from build123d import *

# Parameters (mm, degrees)
SKETCH1_R               = 15
SKETCH1_R_2             = 10
BOSS_EXTRUDE1_DEPTH     = 125
SKETCH2_R               = 15
BOSS_EXTRUDE2_DEPTH     = 40
SKETCH11_W              = 5
SKETCH11_H              = 20
BOSS_EXTRUDE6_DEPTH     = 100
FILLET1_R               = 10
SKETCH12_W              = 28.03455484
SKETCH12_H              = 2
BOSS_EXTRUDE7_DEPTH     = 30
CUT_EXTRUDE1_DEPTH      = 23
CUT_EXTRUDE1_DEPTH_BACK = 5
SKETCH16_R              = 6.25
CUT_EXTRUDE2_DEPTH      = 7


with BuildPart() as part:
    # Sketch1 → Boss-Extrude1 (new body)
    with BuildSketch(Plane.XY):
        Circle(SKETCH1_R)
        Circle(SKETCH1_R_2, mode=Mode.SUBTRACT)
    extrude(amount=BOSS_EXTRUDE1_DEPTH)

    # Sketch2 → Boss-Extrude2 (add)
    with BuildSketch(Plane(origin=(0, 0, 0), x_dir=(1, 0, 0), z_dir=(0, 1, 0))):
        with Locations((0, -62.5)):
            Circle(SKETCH2_R)
    extrude(amount=BOSS_EXTRUDE2_DEPTH)

    # Sketch11 → Boss-Extrude6 (add)
    with BuildSketch(Plane(origin=(0, 0, 0), x_dir=(0, 0, -1), z_dir=(1, 0, 0))):
        with Locations((-62.5, 0)):
            Rectangle(SKETCH11_W, SKETCH11_H)
    extrude(amount=-BOSS_EXTRUDE6_DEPTH)

    # Fillet1
    fillet1_edges = [part.edges().sort_by_distance(p)[0] for p in [
        (-100, -10, 62.5),
        (-100, 10, 62.5),
    ]]
    fillet(fillet1_edges, radius=FILLET1_R - 0.0001)  # a hair under: the kernel refuses the full size

    # Sketch12 → Boss-Extrude7 (add)
    with BuildSketch(Plane(origin=(0, 0, 60), x_dir=(-1, 0, 0), z_dir=(0, 0, -1))):
        with Locations((28.01727742, 0)):
            Rectangle(SKETCH12_W, SKETCH12_H)
    extrude(amount=BOSS_EXTRUDE7_DEPTH)

    # Sketch13 → Cut-Extrude1 (cut, two sides: drawn at the far end of the back side and taken through both)
    with BuildSketch(Plane(origin=(0, 0, 0), x_dir=(1, 0, 0), z_dir=(0, 1, 0)).offset(-CUT_EXTRUDE1_DEPTH_BACK)):
        Polygon((-14.966629547, -30), (-42.03455484, -60), (-42.03455484, -30), align=None)
    extrude(amount=CUT_EXTRUDE1_DEPTH + CUT_EXTRUDE1_DEPTH_BACK, mode=Mode.SUBTRACT)

    # Sketch16 → Cut-Extrude2 (cut)
    with BuildSketch(Plane(origin=(0, 0, 60), x_dir=(-1, 0, 0), z_dir=(0, 0, -1))):
        with Locations((90, 0)):
            Circle(SKETCH16_R)
    extrude(amount=-CUT_EXTRUDE2_DEPTH, mode=Mode.SUBTRACT)


solid = part.part
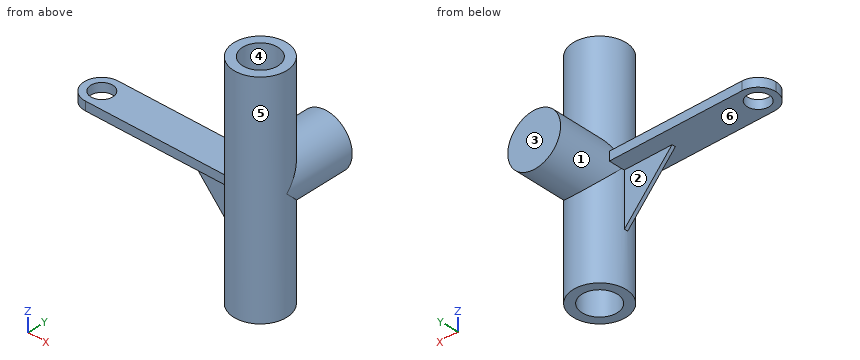
Check sheet for the modelled part. Datum: model origin and axes. Units: mm. Face numbers are marked on the shaded views. A direction names the side the tool comes from. Round coordinates to 2 decimals unless told otherwise and drop trailing zeros. Order: outer loops, then holes, each group sorted by start corner. A loop starts at its lowest first (then second) coordinate and runs counter-clockwise, first axis right, second up.
(1) Access from +Z, -Z, +X, -X, +Y, -Y to the whole of each face (thin tool, end or side, straight path). Record for the marked faces 1, 2 and 3.
(2) Cross-section at C-C, the plane z = 35. Enter the section's corners in (x, y).
(3) Go/stop test with flat-tipped pins: P1, Ø12, axis at y = 19.5, z = 51, coming from the +X side; P2, Ø4, axis at x = -46.5, z = 62.5, coming from the -Y side; P3, Ø10, axis at x = -55.5, y = -1, coming from the -Z side. Record where each tip stops, or that it passes through.
(4) Scan lines: probe 1 along Y at (x, z) = (-90, 62.5); probe 2 along X at (y, z) = (0, 94); probe 3 along Z at (x, y) = (-36, -3). Record each from-to range of solid material in increasing order.
(5) Cross-section at B-B, the plane x = -32. Enter the section's corners in (y, z), and give its area (3 significant figures).
(6) Cross-section at A-A, the plane z = 62.5. State how many separate pieces and enclosed holes the cut face has, and give its area (3 significant figures).
(7) Draft check along Y on the marked faces 4, 5 and 6. Enter one of: pulls with the +Y half, pulls with the -Y half, needs draft (parallel to the pull), parting line crosses it, or undercut.
(8) Cross-section at D-D, the plane y = 30. Enter the section's corners in (x, z), and give its area (3 significant figures).
Check sheet entries:
1. face 1: +Y
1. face 2: -Z, -X, +Y
1. face 3: +Z, -Z, +X, -X, +Y
2. outline: (-19.48, -1) - (-14.97, -1) arc R15 ccw (long way) to (-14.97, 1) - (-19.48, 1) - close; hole circle Ø20 at (0, 0)
3. P1: stops at x = 13.96
3. P2: stops at y = -10
3. P3: stops at z = 60
4. probe 1: y = -10 to -6.25, 6.25 to 10
4. probe 2: x = -15 to -10, 10 to 15
4. probe 3: z = 60 to 65
5. outline: (-10, 60) - (-1, 60) - (-1, 48.88) - (1, 48.88) - (1, 60) - (10, 60) - (10, 65) - (-10, 65) - close
5. area: 122 mm2
6. separate pieces: 1
6. enclosed holes: 2
6. area: 3,020 mm2
7. face 4: undercut
7. face 5: parting line crosses it
7. face 6: needs draft
8. outline: circle Ø30 at (0, 62.5)
8. area: 707 mm2
